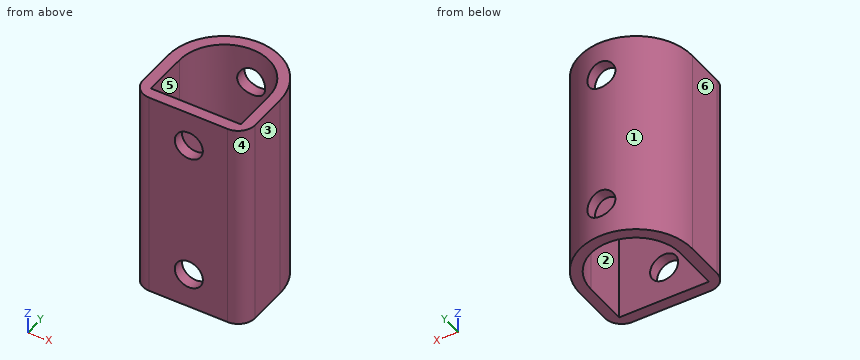
```python
from build123d import *

# Parameters (mm, degrees)
F1_DEPTH      = 75
F3_DEPTH      = 75
F5_R          = 6
F6_R          = 6
F4_R          = 5
F7_DEPTH      = 25
F7_DEPTH_BACK = 36.001


with BuildPart() as f1:
    # F0 (on Top) → F1 (new body)
    with BuildSketch(Plane.XY):
        with BuildLine():
            ThreePointArc((40, 20), (20, 40), (0, 20))
            Line((0, 20), (40, 20))
        make_face()
        with BuildLine():
            ThreePointArc((0, 20), (5.8578643763, 5.8578643763), (20, 0))
            ThreePointArc((20, 0), (34.1421356237, 5.8578643763), (40, 20))
            Line((40, 20), (0, 20))
        make_face()
        with BuildLine():
            ThreePointArc((40, 20), (34.1421356237, 5.8578643763), (20, 0))
            Line((20, 0), (40, 0))
            Line((40, 0), (40, 20))
        make_face()
        with BuildLine():
            Line((0, 20), (0, 0))
            Line((0, 0), (20, 0))
            ThreePointArc((20, 0), (5.8578643763, 5.8578643763), (0, 20))
        make_face()
    extrude(amount=F1_DEPTH)

    # F2 (on face) → F3 (cut)
    with BuildSketch(Plane.XY.offset(75)):
        with BuildLine():
            ThreePointArc((36.1371551045, 20), (20.1371551045, 36), (4.1371551045, 20))
            Line((4.1371551045, 20), (36.1371551045, 20))
        make_face()
        with BuildLine():
            Line((36.1371551045, 20), (4.1371551045, 20))
            ThreePointArc((4.1371551045, 20), (8.8234466055, 8.686291501), (20.1371551045, 4))
            ThreePointArc((20.1371551045, 4), (31.4508636035, 8.686291501), (36.1371551045, 20))
        make_face()
        with BuildLine():
            ThreePointArc((20.1371551045, 4), (8.8234466055, 8.686291501), (4.1371551045, 20))
            Line((4.1371551045, 20), (4.1371551045, 4))
            Line((4.1371551045, 4), (20.1371551045, 4))
        make_face()
        with BuildLine():
            Line((36.1371551045, 4), (36.1371551045, 20))
            ThreePointArc((36.1371551045, 20), (31.4508636035, 8.686291501), (20.1371551045, 4))
            Line((20.1371551045, 4), (36.1371551045, 4))
        make_face()
    extrude(amount=-F3_DEPTH, mode=Mode.SUBTRACT)

    # F5
    f5_edges = [f1.edges().sort_by_distance(p)[0] for p in [
        (40, 0, 37.5),
    ]]
    fillet(f5_edges, radius=F5_R)

    # F6
    f6_edges = [f1.edges().sort_by_distance(p)[0] for p in [
        (0, 0, 37.5),
    ]]
    fillet(f6_edges, radius=F6_R)

    # F4 (on face) → F7 (cut, two sides)
    with BuildSketch(Plane(origin=(0, 4, 0), x_dir=(-1, 0, 0), z_dir=(0, 1, 0))) as f7_sk:
        with Locations((-20.1371551045, 12.5)):
            Circle(F4_R)
        with Locations((-20.1371551045, 62.5)):
            Circle(F4_R)
    extrude(amount=-F7_DEPTH, mode=Mode.SUBTRACT)
    extrude(f7_sk.sketch, amount=F7_DEPTH_BACK, mode=Mode.SUBTRACT)


solid = f1.part
```
For this review, take the finished solid that the model builds, in its own axes (mm). Face numbers are marked on the shaded views. A direction names the side the tool comes from. Coordinates: 2 decimals unless noted, no trailing zeros. Loops run counter-clockwise (first coordinate to the right, second up) from the corner with the lowest first, then second, coordinate; pieces in that order, holes last.
1. Add section D-D, the plane x = 20. Give the boundary of the cut face in (y, z).
2. Add section B-B, the plane z = 62.5. Give the boundary of the cut face in (x, y), then the cut area to 3 significant figures.
3. Add section A-A, the plane y = 11. Give the boundary of the cut face in (x, z).
4. For line 1 (X direction, y = 9, z = 62); line 2 (Z direction, x = 24, y = 2); line 3 (Y direction, x = 10.5, z = 14), list the stretches that pass through material, from the lowest coordinate up.
5. Mouldability with a two-part tool opening along Y and no side actions: class the marked faces 1, 2, 3 and 4 as +Y half, -Y half, draft (parallel to the pull), parting line (faces both ways), or undercut.
6. For the marked faces 5 and 6, list the 3-axis set-ups (+Z, -Z, +X, -X, +Y, -Y) from which the entire face can be reached by the end or side of a thin tool; tool diameter is ignored.
7. Insertion check: P1, Ø12, axis at y = 22, z = 18.5, coming from the +X side; P2, Ø3, axis at x = 13.5, z = 47.5, coming from the +Y side; P3, Ø10, axis at y = 28.5, z = 39.5, coming from the -X side; P4, Ø1.5, axis at y = 33, z = 66, coming from the +X side. Each pin has a flat end and moves straight along its axis. Give the tip position at first contact, or say it passes through.
8. Add section C-C, the plane z = 22. Give the boundary of the cut face in (x, y), then the cut area to 3 significant figures.
Result:
1. outline: (0, 0) - (4, 0) - (4, 7.5) - (0, 7.5) - close; (0, 17.5) - (4, 17.5) - (4, 57.5) - (0, 57.5) - close; (0, 67.5) - (4, 67.5) - (4, 75) - (0, 75) - close; (36, 0) - (40, 0) - (40, 7.5) - (36, 7.5) - close; (36, 17.5) - (40, 17.5) - (40, 57.5) - (36, 57.5) - close; (36, 67.5) - (40, 67.5) - (40, 75) - (36, 75) - close
2. outline: (0, 6) arc R6 ccw to (6, 0) - (15.14, 0) - (15.14, 4) - (4.14, 4) - (4.14, 20) arc R16 cw to (15.14, 35.2) - (15.14, 39.4) arc R20 ccw to (0, 20) - close; (25.14, 0) - (34, 0) arc R6 ccw to (40, 6) - (40, 20) arc R20 ccw to (25.14, 39.33) - (25.14, 35.2) arc R16 cw to (36.14, 20) - (36.14, 4) - (25.14, 4) - close
2. area: 418 mm2
3. outline: (0, 0) - (4.14, 0) - (4.14, 75) - (0, 75) - close; (36.14, 0) - (40, 0) - (40, 75) - (36.14, 75) - close
4. line 1: x = 0 to 4.14, 36.14 to 40
4. line 2: z = 0 to 9.33, 15.67 to 59.33, 65.67 to 75
4. line 3: y = 0 to 4, 32.77 to 37.6
5. face 1: +Y half
5. face 2: undercut
5. face 3: draft
5. face 4: -Y half
6. face 5: +Z, -Z
6. face 6: +Z, -Z, -X, +Y, -Y
7. P1: stops at x = 40
7. P2: stops at y = 39.36
7. P3: stops at x = 0.31
7. P4: stops at x = 35.81
8. outline: (0, 6) arc R6 ccw to (6, 0) - (34, 0) arc R6 ccw to (40, 6) - (40, 20) arc R20 ccw to (0, 20) - close; hole (4.14, 4) - (36.14, 4) - (36.14, 20) arc R16 ccw to (4.14, 20) - close
8. area: 499 mm2
